Geometry check sheet. Reference: the model listing, model coordinates, mm. Round coordinates to 2 decimals unless told otherwise and drop trailing zeros. Loops run counter-clockwise (first coordinate to the right, second up) from the corner with the lowest first, then second, coordinate; pieces in that order, holes last. Notation, with made-up numbers: (16.25, 18) - (75.25, 18) arc R13 ccw to (75.25, 26) - close; hole circle Ø8 at (51.5, 35.5). An arc over 180 degrees is marked (long way). Answer as CSV lines item,"result". Start each with the question number.
1) Cross-section at D-D on y = 29. Record the boundary of the cut face in (x, z), and give its area (3 significant figures).
2) Cross-section at A-A on y = 18.77. Record the boundary of the cut face in (x, z) (3 decimals).
3) Draft check along Y on faces 1 (the cylindrical face through (0.493, 37.571, 6.436)), 2 (the conical face through (0.635, 17.497, -17.483)), 3 (the cylindrical face through (0.49, 1.2, 23.65)), 4 (the flat face through (0.493, 35.177, -10.57)). Enter one of: released by +Y, released by -Y, zero draft, split by the parting line, or undercut.
4) Thickness scan on line 1 along Y through (x, z) = (0.9, 5.5); line 2 along Z through (x, y) = (0.8, 3.5); line 3 along Y through (x, z) = (0.85, -20.5). Record the ranges inside material, lowest first.
5) Cross-section at C-C on z = -7. Record the boundary of the cut face in (x, y), and give its area (3 significant figures).
6) Cross-section at B-B on x = 0.2. Record the boundary of the cut face in (y, z).
7) Depth check by flat-ended pin: P1, Ø0.6, axis at x = 0, y = 4.5, coming from the -Z side; P2, Ø1.6, axis at y = 18.5, z = -19, coming from the +X side; P3, Ø0.6, axis at x = 0, y = 5.5, coming from the +Z side; P4, Ø1.1, axis at y = 4, z = 18.5, coming from the +X side. Enter the tip coordinate at first touch or a pass-through.
from build123d import *

# Parameters (mm, degrees)
SKETCH1_R           = 3.65
SKETCH1_W           = 3
SKETCH1_H           = 3
SKETCH1_W_2         = 2.35
SKETCH1_H_2         = 2.46
BOSS_EXTRUDE1_DEPTH = 1
SKETCH3_R           = 2.09
CUT_EXTRUDE1_DEPTH  = 0.5
CUT_EXTRUDE1_TAPER  = 30


with BuildPart() as part:
    # Sketch1 → Boss-Extrude1 (new body)
    with BuildSketch(Plane(origin=(0, 0, 0), x_dir=(0, 0, -1), z_dir=(1, 0, 0))):
        with BuildLine():
            Line((-20.402250922, 0), (20.402250922, 0))
            ThreePointArc((20.402250922, 0), (23.937784828, 1.464466094), (25.402250922, 5))
            Line((25.402250922, 5), (25.402250922, 21.50709196))
            ThreePointArc((25.402250922, 21.50709196), (24.87692273, 23.738081025), (23.411326038, 25.50026951))
            Line((23.411326038, 25.50026951), (-2.635195634, 45.127731407))
            ThreePointArc((-2.635195634, 45.127731407), (-6.321071977, 46.088536103), (-9.61416456, 44.174281334))
            Line((-9.61416456, 44.174281334), (-26.788641191, 21.74435991))
            ThreePointArc((-26.788641191, 21.74435991), (-27.676067974, 19.890565251), (-27.742786146, 17.836391544))
            Line((-27.742786146, 17.836391544), (-25.326289687, 4.131759112))
            ThreePointArc((-25.326289687, 4.131759112), (-23.61618897, 1.169777784), (-20.402250922, 0))
        make_face()
        with Locations((-5.64427075, 41.134553857)):
            Circle(SKETCH1_R, mode=Mode.SUBTRACT)
        with Locations((19.19182941, 19.04)):
            Rectangle(SKETCH1_W, SKETCH1_H, mode=Mode.SUBTRACT)
        with Locations((18.865, 5)):
            Rectangle(SKETCH1_W_2, SKETCH1_H_2, mode=Mode.SUBTRACT)
        with Locations((-18.865, 5)):
            Rectangle(SKETCH1_W_2, SKETCH1_H_2, mode=Mode.SUBTRACT)
    extrude(amount=BOSS_EXTRUDE1_DEPTH)

    # Sketch3 → Cut-Extrude1 (cut)
    with BuildSketch(Plane(origin=(1, 0, 0), x_dir=(0, 0, -1), z_dir=(1, 0, 0))):
        with Locations((-18.865, 5)):
            Circle(SKETCH3_R)
        with Locations((18.865, 5)):
            Circle(SKETCH3_R)
        with Locations((18.865, 18.77)):
            Circle(SKETCH3_R)
    extrude(amount=-CUT_EXTRUDE1_DEPTH, taper=CUT_EXTRUDE1_TAPER, mode=Mode.SUBTRACT)


solid = part.part
Answer block:
1,outline,"(0, -18.77) - (1, -18.77) - (1, 21.23) - (0, 21.23) - close"
1,area,"40.0 mm^2"
2,outline,"(0, -25.402) - (1, -25.402) - (1, -20.955) - (0.544, -20.692) - (0, -20.692) - close; (0, -17.692) - (0.5, -17.692) - (0.5, -17.064) - (1, -16.775) - (1, 27.818) - (0, 27.818) - close"
3,face 1,"undercut"
3,face 2,"undercut"
3,face 3,"released by -Y"
3,face 4,"released by +Y"
4,line 1,"y = 0 to 37.49, 44.78 to 46.13"
4,line 2,"z = -25.17 to -20.15, -17.58 to 17.58, 20.15 to 25.17"
4,line 3,"y = 0 to 3.84, 6.16 to 17.54, 20.54 to 27.69"
5,outline,"(0, 0) - (1, 0) - (1, 37.87) - (0, 37.87) - close"
5,area,"37.9 mm^2"
6,outline,"(0, -20.4) arc R5 ccw to (5, -25.4) - (21.51, -25.4) arc R5 ccw to (25.5, -23.41) - (45.13, 2.64) arc R5 ccw to (44.17, 9.61) - (21.74, 26.79) arc R5 ccw to (17.84, 27.74) - (4.13, 25.33) arc R5 ccw to (0, 20.4) - close; hole (3.77, -20.04) - (6.23, -20.04) - (6.23, -17.69) - (3.77, -17.69) - close; hole (3.77, 17.69) - (6.23, 17.69) - (6.23, 20.04) - (3.77, 20.04) - close; hole (17.54, -20.69) - (20.54, -20.69) - (20.54, -17.69) - (17.54, -17.69) - close; hole circle Ø7.3 at (41.13, 5.64)"
7,P1,"stops at z = -25.4"
7,P2,"passes through"
7,P3,"stops at z = 25.62"
7,P4,"stops at x = 0.5"
